Design review of the part built by this model. Coordinates are the model's own, in mm. Round coordinates to 2 decimals unless told otherwise and drop trailing zeros. Loops run counter-clockwise (first coordinate to the right, second up) from the corner with the lowest first, then second, coordinate; pieces in that order, holes last. Notation, with made-up numbers: (71, -14.5) -> (123, -14.5) arc R4 cw to (123, -9.5) -> close; hole circle Ø8 at (33.5, 72). An arc over 180 degrees is marked (long way). Answer as CSV lines item,"result". Start each with the question number.
(1) Take a section at C-C, the plane y = 1.35. Write out the cut boundary in (x, z).
(2) Take a section at D-D, the plane y = -0.95. Write out the cut boundary in (x, z).
(3) For P1, Ø1.5, axis at x = 5.5, y = -1, coming from the -Z side; P2, Ø1, axis at y = 1, z = 7, coming from the +X side, all flat-tipped, find the tip position at first contact; note any pin that passes through.
(4) To check wall thickness, follow line 1 (Z direction, x = 14.75, y = 0.1); line 2 (X direction, y = -0.1, z = 5.5); line 3 (Y direction, x = 9.25, z = -18). State the ranges of each line that lie inside material, in increasing order. Write a range as from..to.
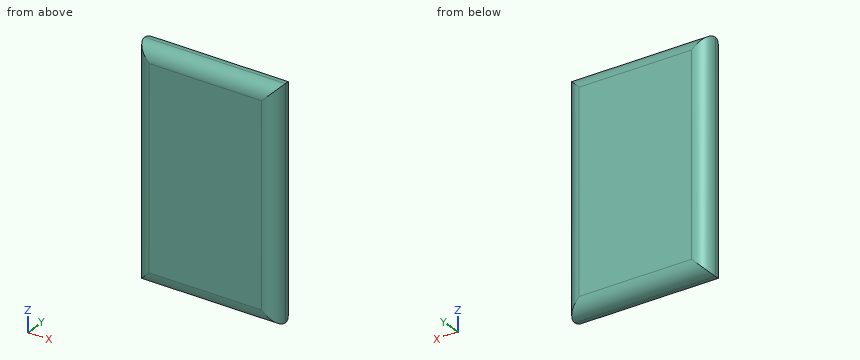
from build123d import *

# Parameters (mm, degrees)
SKETCH2_W           = 40.64
SKETCH2_H           = 5.08
BOSS_EXTRUDE1_DEPTH = 25.4
FILLET1_R           = 2.54


with BuildPart() as part:
    # Sketch2 → Boss-Extrude1 (new body)
    with BuildSketch(Plane(origin=(0, 0, 0), x_dir=(0, 0, -1), z_dir=(1, 0, 0))):
        Rectangle(SKETCH2_W, SKETCH2_H)
    extrude(amount=BOSS_EXTRUDE1_DEPTH)

    # Fillet1
    fillet1_edges = [part.edges().sort_by_distance(p)[0] for p in [
        (12.7, -2.54, 20.32),
        (25.4, -2.54, 0),
        (12.7, -2.54, -20.32),
        (0, -2.54, 0),
        (12.7, 2.54, -20.32),
        (25.4, 2.54, 0),
        (12.7, 2.54, 20.32),
        (0, 2.54, 0),
    ]]
    fillet(fillet1_edges, radius=FILLET1_R - 0.0001)  # a hair under: the kernel refuses the full size


solid = part.part
The answers:
1,outline,"(0.39, -19.93) -> (25.01, -19.93) -> (25.01, 19.93) -> (0.39, 19.93) -> close"
2,outline,"(0.18, -20.14) -> (25.22, -20.14) -> (25.22, 20.14) -> (0.18, 20.14) -> close"
3,P1,"z = -20.31"
3,P2,"x = 25.35"
4,line 1,"-20.32..20.32"
4,line 2,"0..25.4"
4,line 3,"-2.53..2.53"
